For this review, take the finished solid that the model builds, in its own axes (mm). Face numbers are marked on the shaded views. A direction names the side the tool comes from. Round coordinates to 2 decimals unless told otherwise and drop trailing zeros. Order: outer loops, then holes, each group sorted by start corner. A loop starts at its lowest first (then second) coordinate and runs counter-clockwise, first axis right, second up. Notation, with made-up numbers: M 55.25,56.25 L 61.25,56.25 A12 ccw 61.25,68.25 Z; hole C 21.5,54.5 d2. An arc over 180 degrees is marked long. Use a Markdown table: item, result.
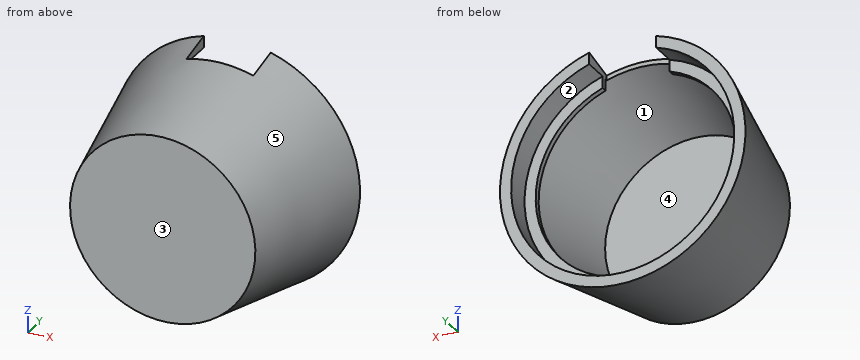
from build123d import *

# Parameters (mm, degrees)
SKETCH_2_W          = 60
SKETCH_2_H          = 57.613168724
CUT_EXTRUDE_1_DEPTH = 30


with BuildPart() as part:
    # 草圖1 → 旋轉1 (revolve)
    with BuildSketch(Plane(origin=(0, 0, 0), x_dir=(0, 0, -1), z_dir=(1, 0, 0)), mode=Mode.PRIVATE) as revolve_1_sk:
        Polygon((0, 0), (83.034457175, 0), (110, 128), (100, 128), (100, 105), (90, 105), (90, 100), (100.013488815, 100), (80, 5), (0, 5), align=None)
    revolve(revolve_1_sk.sketch.rotate(Axis((0, 5, 0), (0, -1, 0)), 180), axis=Axis((0, 5, 0), (0, -1, 0)))

    # 草圖2 → 除料-伸長1 (cut)
    with BuildSketch(Plane(origin=(0, 128, 0), x_dir=(1, 0, 0), z_dir=(0, 1, 0))):
        with Locations((0, -98.621202087)):
            Rectangle(SKETCH_2_W, SKETCH_2_H)
    extrude(amount=-CUT_EXTRUDE_1_DEPTH, mode=Mode.SUBTRACT)


solid = part.part
Q1. Draft analysis for pull direction X (two halves, no side actions). For the marked faces 3, 4 and 5, state which applies: pulls with the +X half, pulls with the -X half, needs draft (parallel to the pull), parting line crosses it, or undercut.
Determined:
| item | result |
|---|---|
| face 3 | needs draft |
| face 4 | undercut |
| face 5 | parting line crosses it |
Q2. Add section D-D (y = 118.5). Write out the cut boundary in (x, z), then the cut area to 3 significant figures.
Determined:
| item | result |
|---|---|
| outline | M -30,95.39 L -30,103.75 A108 ccw long 30,103.75 L 30,95.39 A100 cw long Z |
| area | 4,740 mm^2 |
Q3. Add section B-B (x = 0). Write out the cut boundary in (y, z), then the cut area to 3 significant figures.
Determined:
| item | result |
|---|---|
| outline | M 0,-83.03 L 128,-110 L 128,-100 L 105,-100 L 105,-90 L 100,-90 L 100,-100.01 L 5,-80 L 5,80 L 98,99.59 L 98,103.68 L 0,83.03 Z |
| area | 1,850 mm^2 |
Q4. Add section A-A (z = 0). Write out the cut boundary in (x, y), then the cut area to 3 significant figures.
Determined:
| item | result |
|---|---|
| outline | M -110,128 L -83.03,0 L 83.03,0 L 110,128 L 100,128 L 100,105 L 90,105 L 90,100 L 100.01,100 L 80,5 L -80,5 L -100.01,100 L -90,100 L -90,105 L -100,105 L -100,128 Z |
| area | 2,110 mm^2 |
Q5. Add section C-C (y = 43). Write out the cut boundary in (x, z), then the cut area to 3 significant figures.
Determined:
| item | result |
|---|---|
| outline | C 0,0 d184.19; hole C 0,0 d176.01 |
| area | 2,310 mm^2 |
Q6. Clearance check with flat-ended pins moving along their axes: pin 1 (3 mm diameter, centred on y = 72, z = 53.5, fed in from +X); pin 2 (4 mm diameter, centred on x = 69, y = 16, fed in from -Z); pin 3 (5 mm diameter, centred on y = 53.5, z = 34.5, fed in from -X). State where each tip first meets the part, or that it passes through.
Determined:
| item | result |
|---|---|
| pin 1 | stops at x = 83.38 |
| pin 2 | stops at z = -54.65 |
| pin 3 | stops at x = -88.87 |
Q7. Wall thickness on line 1 along Z through (x, y) = (-87, 96); line 2 along X through (y, z) = (63.5, -14); line 3 along X through (y, z) = (96, 91.5): over which ranges is each line inside the solid? List them lowest first. Write a range as [from, to].
Determined:
| item | result |
|---|---|
| line 1 | z = [-55.62, -47.6], [47.6, 55.62] |
| line 2 | x = [-95.39, -91.26], [91.26, 95.39] |
| line 3 | x = [-47.85, -38.24], [38.24, 47.85] |
Q8. Machinability: for the marked faces 1 and 2, which of the approach directions +Z, -Z, +X, -X, +Y, -Y give a long, thin tool a straight path to every point of the face, cutting with its end or side? Answer none if there is none.
Determined:
| item | result |
|---|---|
| face 1 | none |
| face 2 | +Y |
